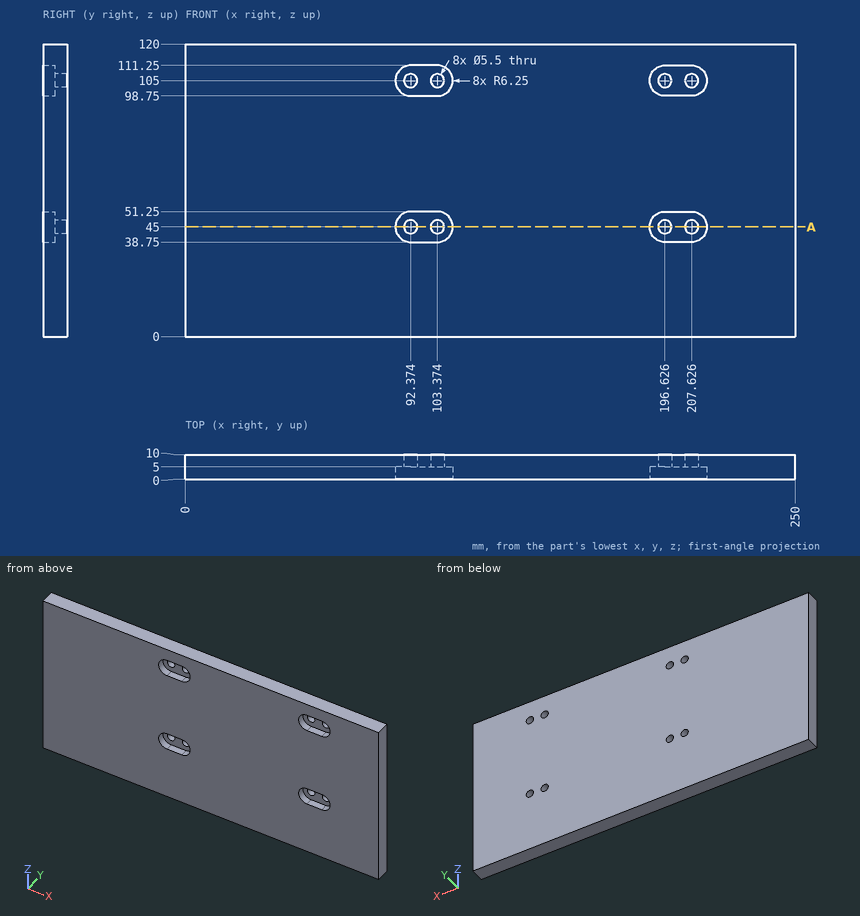
Can you work these out from the drawing? Everything is in mm from the part's minimum corner. Coordinates: 2 decimals unless noted, no trailing zeros. Write each loop counter-clockwise with the first axis right and the second up, starting at its lowest first coordinate (ties: lowest second). Pieces come first, ordered by that corner, then holes. Notation, with made-up numbers: (5, -31.5) -> (30, -31.5) arc R9 ccw to (30, -21.5) -> close; hole circle Ø5 at (24, 50). An arc over 180 degrees is marked (long way). Write each question's results on one line, items separated by ' | '. Start each with the question number.
Q1. Imagine slicing it at A-A (z = 45). Write out the boundary of the cut face in (x, y) (1 decimal).
Q2. I'm going to push flat-ended pins straight in: pin 1 (5.5 mm diameter, centred on x = 201, y = 2.5, fed in from -Z); pin 2 (3.5 mm diameter, centred on x = 196.63, z = 105, fed in from +Y); pin 3 (6 mm diameter, centred on x = 197.5, z = 105, fed in from -Y). Where does each tip first touch, or does it pass through?
Q3. If I drill on probe 1 along X at (y, z) = (2.75, 102), over which ranges is the centre line in solid material (lowest first)?
Taken from the geometry:
1) outline: (0, 0) -> (86.1, 0) -> (86.1, 5) -> (89.6, 5) -> (89.6, 10) -> (0, 10) -> close; (95.1, 5) -> (100.6, 5) -> (100.6, 10) -> (95.1, 10) -> close; (106.1, 5) -> (109.6, 5) -> (109.6, 0) -> (190.4, 0) -> (190.4, 5) -> (193.9, 5) -> (193.9, 10) -> (106.1, 10) -> close; (199.4, 5) -> (204.9, 5) -> (204.9, 10) -> (199.4, 10) -> close; (210.4, 5) -> (213.9, 5) -> (213.9, 0) -> (250, 0) -> (250, 10) -> (210.4, 10) -> close
2) pin 1: stops at z = 0 | pin 2: passes through | pin 3: stops at y = 5
3) probe 1: x = 0 to 86.89, 108.86 to 191.14, 213.11 to 250
